Geometry check sheet. Reference: the model listing, model coordinates, mm. Face numbers are marked on the shaded views. A direction names the side the tool comes from. Round coordinates to 2 decimals unless told otherwise and drop trailing zeros. Order: outer loops, then holes, each group sorted by start corner. A loop starts at its lowest first (then second) coordinate and runs counter-clockwise, first axis right, second up.
(1) Sectioned sample at B-B (y = 8.75). Record the boundary of the cut face in (x, z).
(2) Go/stop test with flat-tipped pins: pin 1 (1.2 mm diameter, centred on x = 10.5, y = -1, fed in from +Z); pin 2 (10 mm diameter, centred on x = 10, y = 4, fed in from +Z); pin 3 (8.5 mm diameter, centred on x = 2, z = 4.5, fed in from -Y). Record where each tip stops, or that it passes through.
(3) Set-up check for the marked faces 4, 5, 6 and 7: record each of +Z, -Z, +X, -X, +Y, -Y from which the full face is reachable in a straight line by a thin tool's end or side.
(4) Sectioned sample at A-A (x = -8.5). Record the boundary of the cut face in (y, z), plus the area to 3 significant figures.
(5) Material ranges on line 1 along Z through (x, y) = (6.75, 2.25); line 2 along X through (y, z) = (-1.5, 10); line 3 along Z through (x, y) = (-9.75, -9), recorded low to high.
(6) Sectioned sample at C-C (z = 9). Record the boundary of the cut face in (x, y).
(7) Release check for a two-part mould opening along Z. For the marked faces 1, 2 and 3 record: +Z half, -Z half, draft (parallel to the pull), parting line (faces both ways), or undercut.
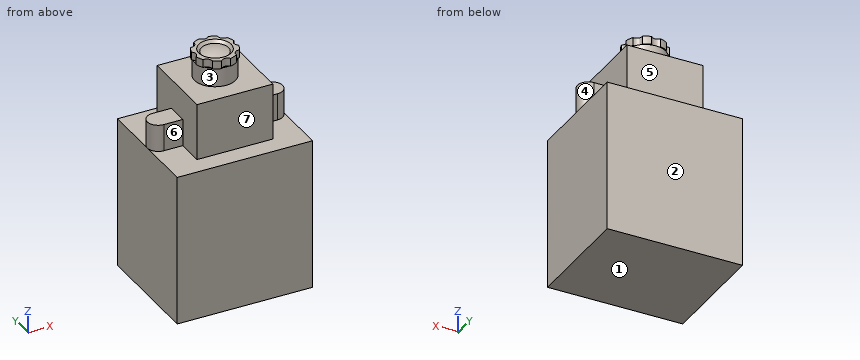
from build123d import *
from build123d.topology import SkipClean

# Parameters (mm, degrees)
SKETCH_1_W               = 14
SKETCH_1_H               = 14
EXTRUDE_1_DEPTH          = 10.5
SKETCH_2_R               = 3.8
EXTRUDE_2_DEPTH          = 5
SKETCH_3_R               = 4
EXTRUDE_3_DEPTH          = 1.5
SKETCH_4_R               = 1
CUT_EXTRUDE_2_DEPTH      = 1.5
PATTERN_CIRCULAR_1_COUNT = 8
SKETCH_5_W               = 25
SKETCH_5_H               = 21
EXTRUDE_4_DEPTH          = 28
EXTRUDE_5_DEPTH          = 5
SKETCH_9_R               = 3
CUT_EXTRUDE_3_DEPTH      = 0.5
CHAMFER_1_SIZE           = 0.5


with BuildPart() as part:
    # 草圖1 → 填料-伸長1 (new body)
    with BuildSketch(Plane.XY):
        Rectangle(SKETCH_1_W, SKETCH_1_H)
    extrude(amount=EXTRUDE_1_DEPTH)

    # 草圖2 → 填料-伸長2 (add)
    with BuildSketch(Plane.XY.offset(10.5)):
        Circle(SKETCH_2_R)
    extrude(amount=EXTRUDE_2_DEPTH)

    # 草圖3 → 填料-伸長3 (add)
    with BuildSketch(Plane.XY.offset(15.5)):
        Circle(SKETCH_3_R)
    extrude(amount=-EXTRUDE_3_DEPTH)

    # 草圖4 → 除料-伸長2 (cut)
    with BuildSketch(Plane.XY.offset(15.5)):
        with Locations((0, 4.5)):
            Circle(SKETCH_4_R)
    cut_extrude_2 = extrude(amount=-CUT_EXTRUDE_2_DEPTH, mode=Mode.SUBTRACT)

    # 環狀複製排列1: 除料-伸長2 ×8 about axis
    pattern_circular_1_axis = Axis((0, 0, 0), (0, 0, 1))
    for i in range(1, PATTERN_CIRCULAR_1_COUNT):
        add(cut_extrude_2.rotate(pattern_circular_1_axis, i * 360 / PATTERN_CIRCULAR_1_COUNT), mode=Mode.SUBTRACT)

    # 草圖5 → 填料-伸長4 (add)
    with BuildSketch(Plane(origin=(0, 0, 0), x_dir=(-1, 0, 0), z_dir=(0, 0, -1))):
        Rectangle(SKETCH_5_W, SKETCH_5_H)
    extrude(amount=EXTRUDE_4_DEPTH)

    # 草圖6 → 填料-伸長5 (add)
    with BuildSketch(Plane.XY):
        with BuildLine():
            Line((-7, -2), (-7, 2))
            Line((-7, 2), (-10.5, 2))
            ThreePointArc((-10.5, 2), (-12.5, 0), (-10.5, -2))
            Line((-10.5, -2), (-7, -2))
        make_face()
    extrude_5 = extrude(amount=EXTRUDE_5_DEPTH)

    # 鏡射1: 填料-伸長5 across plane
    add(extrude_5.mirror(Plane(origin=(0, 0, 0), x_dir=(0, 0, 1), z_dir=(1, 0, 0))))

    # 草圖9 → 除料-伸長3 (cut)
    with BuildSketch(Plane.XY.offset(15.5)):
        Circle(SKETCH_9_R)
    extrude(amount=-CUT_EXTRUDE_3_DEPTH, mode=Mode.SUBTRACT)

    # 導角1
    chamfer_1_edges = [part.edges().sort_by_distance(p)[0] for p in [
        (-3, 0, 15),
    ]]
    chamfer(chamfer_1_edges, length=CHAMFER_1_SIZE - 0.0001)  # a hair under: the kernel refuses the full size

    # 草圖10 → 旋轉2 (revolve)
    with SkipClean():  # the faces are left unmerged after this step: merging them gives an invalid solid
        with BuildSketch(Plane(origin=(0, 0, 0), x_dir=(1, 0, 0), z_dir=(0, 1, 0)), mode=Mode.PRIVATE) as revolve_2_sk:
            with BuildLine():
                Line((2.5, -15), (0, -15))
                Line((0, -15), (0, -15.5))
                ThreePointArc((0, -15.5), (1.274754878, -15.373774392), (2.5, -15))
            make_face()
            with BuildLine():
                Line((0, -15.5), (0, -15))
                Line((0, -15), (-2.5, -15))
                ThreePointArc((-2.5, -15), (-1.274754878, -15.373774392), (0, -15.5))
            make_face()
        revolve(revolve_2_sk.sketch.rotate(Axis((0, 0, 0), (0, 0, 1)), 170.092802055), axis=Axis((0, 0, 0), (0, 0, 1)))
    add(part.part.scale(1), mode=Mode.REPLACE)  # the faces are merged on a copy


solid = part.part
Answer below:
1. outline: (-12.5, -28) - (12.5, -28) - (12.5, 0) - (-12.5, 0) - close
2. pin 1: stops at z = 5
2. pin 2: stops at z = 10.5
2. pin 3: stops at y = -7
3. face 4: +Z, +X
3. face 5: +Z, +X, -X, +Y
3. face 6: +Z, -X, -Y
3. face 7: +Z, +X, -X, -Y
4. outline: (-10.5, -28) - (10.5, -28) - (10.5, 0) - (2, 0) - (2, 5) - (-2, 5) - (-2, 0) - (-10.5, 0) - close
4. area: 608 mm2
5. line 1: z = -28 to 10.5
5. line 2: x = -7 to 7
5. line 3: z = -28 to 0
6. outline: (-7, -7) - (7, -7) - (7, 7) - (-7, 7) - close
7. face 1: -Z half
7. face 2: draft
7. face 3: undercut
